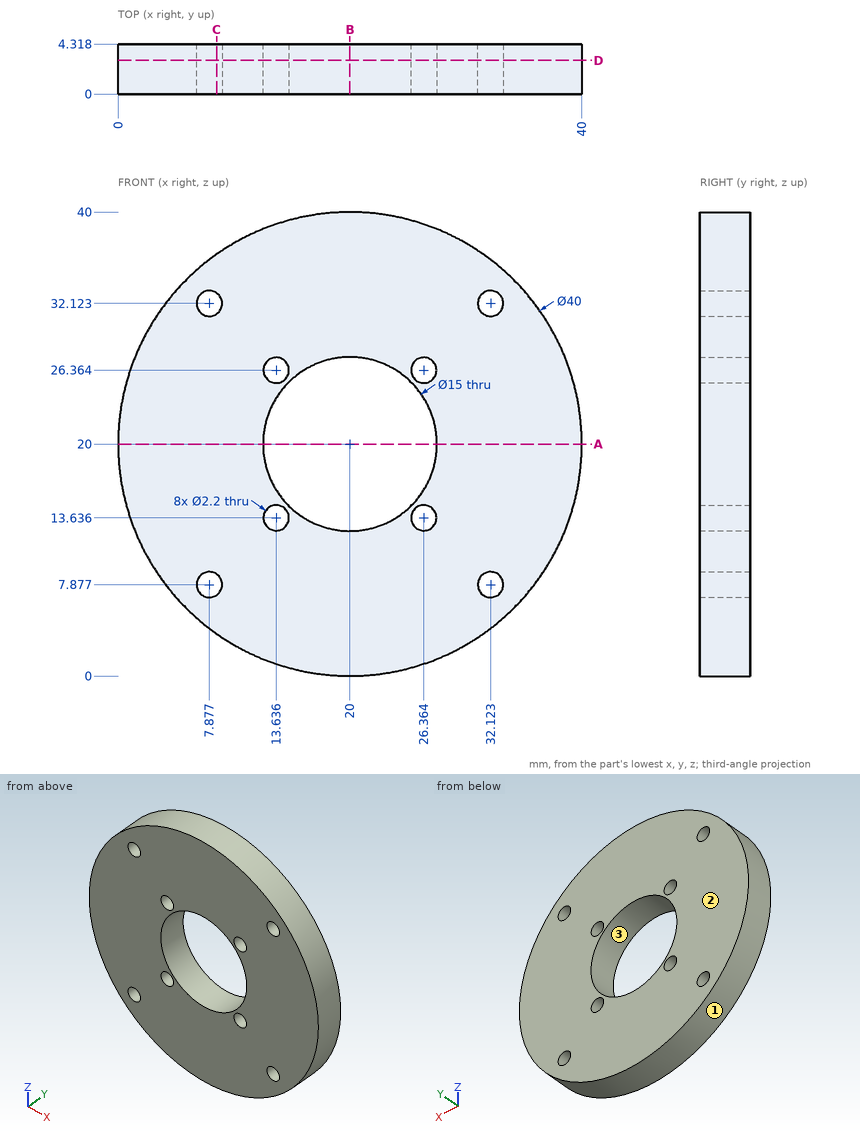
Source: three-view drawing plus pictorial views. Frame: mm from the lowest corner of the part. Round coordinates to 2 decimals unless told otherwise and drop trailing zeros. Loops run counter-clockwise (first coordinate to the right, second up) from the corner with the lowest first, then second, coordinate; pieces in that order, holes last.
Q1. Section C-C on x = 8.5. Return loops of the section in (y, z), plus the area to 3 significant figures.
Q2. Section B-B on x = 20. Return loops of the section in (y, z).
Q3. Material intervals for L1, parallel to Z at x = 24.5, y = 0.65; L2, parallel to Z at x = 21, y = 1.2 (1 decimal), sorted ascending.
Q4. Section D-D on y = 2.9. State how many separate pieces and enclosed holes the cut face has, plus the area to 3 significant figures.
Q5. Section A-A on z = 20. Return loops of the section in (x, y).
Q6. Pin query (flat end, axial travel): P1, Ø1.8, axis at x = 7.88, z = 7.88, coming from the +Y side; P2, Ø1, axis at x = 6, y = 3, coming from the +Z side; P3, Ø2, axis at x = 22.5, y = 1, coming from the -Z side; P4, Ø2, axis at x = 8, y = 2.5, coming from the +Z side. Return the tip coordinate at first contact, or that it passes through.
Q7. Pull-direction query (X, two-part tool) for the marked faces 1, 2 and 3; classes: released by +X, released by -X, zero draft, split by the parting line, or undercut.
Evaluation:
1. outline: (0, 3.64) - (4.32, 3.64) - (4.32, 6.97) - (0, 6.97) - close; (0, 8.78) - (4.32, 8.78) - (4.32, 31.22) - (0, 31.22) - close; (0, 33.03) - (4.32, 33.03) - (4.32, 36.36) - (0, 36.36) - close
1. area: 126 mm2
2. outline: (0, 0) - (4.32, 0) - (4.32, 12.5) - (0, 12.5) - close; (0, 27.5) - (4.32, 27.5) - (4.32, 40) - (0, 40) - close
3. L1: z = 0.51 to 14, 26 to 39.49
3. L2: z = 0 to 12.6, 27.4 to 40
4. separate pieces: 1
4. enclosed holes: 9
4. area: 1,050 mm2
5. outline: (0, 0) - (12.5, 0) - (12.5, 4.32) - (0, 4.32) - close; (27.5, 0) - (40, 0) - (40, 4.32) - (27.5, 4.32) - close
6. P1: passes through
6. P2: stops at z = 34.76
6. P3: stops at z = 0.06
6. P4: stops at z = 36.7
7. face 1: split by the parting line
7. face 2: zero draft
7. face 3: undercut
